Design review of the part built by this model. Coordinates are the model's own, in mm. Face numbers are marked on the shaded views. A direction names the side the tool comes from. Give positions to 0.01 mm unless a question says otherwise; leave off trailing zeros. Loops run counter-clockwise (first coordinate to the right, second up) from the corner with the lowest first, then second, coordinate; pieces in that order, holes last. Notation, with made-up numbers: M 19.25,61 L 29.25,61 A9 cw 29.25,71 Z; hole C 17,6 d1. An arc over 180 degrees is marked long. Use one line per item in the form item = value. Start each with the question number.
from build123d import *

# Parameters (mm, degrees)
F0_R          = 50
F1_DEPTH      = 5
F2_R          = 30
F3_DEPTH      = 10
F4_R          = 24.95
F5_DEPTH      = 6
F6_W          = 13.7062855065
F6_H          = 30
F7_DEPTH      = 100
F7_DEPTH_BACK = 10
F8_SIZE       = 1


with BuildPart() as f1:
    # F0 (on Top) → F1 (new body)
    with BuildSketch(Plane.XY):
        Circle(F0_R)
    extrude(amount=F1_DEPTH)

    # F2 (on face) → F3 (join)
    with BuildSketch(Plane.XY.offset(5)):
        Circle(F2_R)
    extrude(amount=F3_DEPTH)

    # F4 (on face) → F5 (join)
    with BuildSketch(Plane.XY.offset(15)):
        Circle(F4_R)
    extrude(amount=F5_DEPTH)

    # F6 (on Right) → F7 (cut, two sides)
    with BuildSketch(Plane.YZ) as f7_sk:
        with Locations((0, 21)):
            Rectangle(F6_W, F6_H)
    extrude(amount=-F7_DEPTH, mode=Mode.SUBTRACT)
    extrude(f7_sk.sketch, amount=F7_DEPTH_BACK, mode=Mode.SUBTRACT)

    # F8
    f8_edges = [f1.edges().sort_by_distance(p)[0] for p in [
        (24.95, 0, 21),
    ]]
    chamfer(f8_edges, length=F8_SIZE)


solid = f1.part
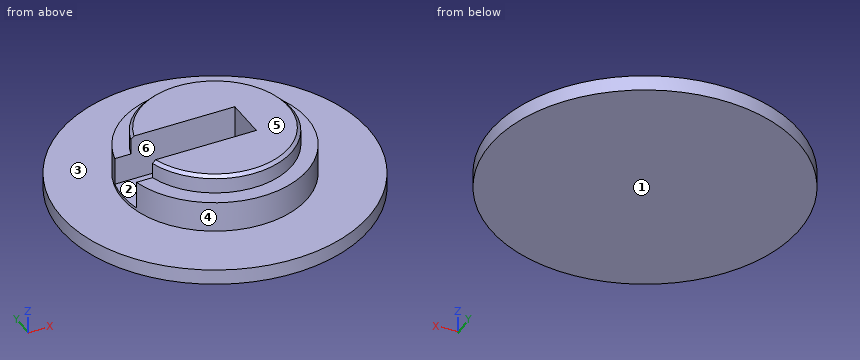
Q1. For the marked faces 1, 2 and 3, list the 3-axis set-ups (+Z, -Z, +X, -X, +Y, -Y) from which the entire face can be reached by the end or side of a thin tool; tool diameter is ignored.
Q2. Clearance check with flat-ended pins moving along their axes: pin 1 Ø10 at (y, z) = (-15, 4.5) entering from +X; pin 2 Ø10 at (x, z) = (1, 13) entering from +Y; pin 3 Ø3 at (y, z) = (25.5, 12.5) entering from -X. State where each tip first meets the part, or that it passes through.
Q3. Take a section at D-D on x = -38. Give the boundary of the cut face in (y, z).
Q4. Take a section at A-A on x = 0. Give the boundary of the cut face in (y, z).
Q5. Take a section at B-B on z = 1.75. Give the boundary of the cut face in (x, y).
Q6. The part is to be moulded in two halves that separate along Y. For the marked faces 4, 5 and 6, say which applies: pulls with the +Y half, pulls with the -Y half, needs draft (parallel to the pull), parting line crosses it, or undercut.
Q7. Take a section at C-C on z = 18.75. Give the boundary of the cut face in (x, y).
Q8. Wall thickness on probe 1 along Y at (x, z) = (-7, 15.5); probe 2 along Z at (x, y) = (7.5, 24); probe 3 along Z at (x, y) = (-28.5, -37): over which ranges is each line inside the solid? List them lowest first.
Response values:
q1.face_1 = -Z, +X, -X, +Y, -Y
q1.face_2 = +Z, -X
q1.face_3 = +Z
q2.pin_1 = 48.99
q2.pin_2 = 30
q2.pin_3 = -18
q3.outline = M -32.5,0 L 32.5,0 L 32.5,5 L -32.5,5 Z
q4.outline = M -50,0 L 50,0 L 50,5 L 30,5 L 30,15 L 24.95,15 L 24.95,20 L 23.95,21 L 6.85,21 L 6.85,6 L -6.85,6 L -6.85,21 L -23.95,21 L -24.95,20 L -24.95,15 L -30,15 L -30,5 L -50,5 Z
q5.outline = C 0,0 d100
q6.face_4 = parting line crosses it
q6.face_5 = needs draft
q6.face_6 = undercut
q7.outline = M -23.99,-6.85 A24.95 ccw long -23.99,6.85 L 10,6.85 L 10,-6.85 Z
q8.probe_1 = -23.95 to -6.85, 6.85 to 23.95
q8.probe_2 = 0 to 15
q8.probe_3 = 0 to 5
